Geometry check sheet. Reference: drawing and pictorial views, mm from the part's lowest x, y, z. Give positions to 0.01 mm unless a question says otherwise; leave off trailing zeros. Write each loop counter-clockwise with the first axis right and the second up, starting at its lowest first coordinate (ties: lowest second). Pieces come first, ordered by that corner, then holes. Notation, with made-up numbers: (43, -16.75) - (88, -16.75) arc R28 ccw to (88, 11.25) - close; hole circle Ø5 at (27, 15). An arc over 180 degrees is marked (long way). Write item = value, one per line. Start each with the question number.
(1) Section check A-A, the plane x = 3.5. Enter the section's corners in (y, z).
(2) Section check B-B, the plane z = 6. Enter the section's corners in (x, y).
(3) Section check C-C, the plane y = 1. Enter the section's corners in (x, z).
(4) Thickness scan on L1, parallel to Y at x = 3.5, z = 9; L2, parallel to X at y = 4, z = 33 (1 decimal); L3, parallel to X at y = 4.25, z = 20.5 (1 decimal). Record the ranges inside material, lowest first.
(5) Depth check by flat-ended pin: pin 1 Ø3 at (x, y) = (1.5, 3) entering from -Z; pin 2 Ø1.8 at (x, y) = (3.5, 3.03) entering from +Z. Enter the tip coordinate at first touch or a pass-through.
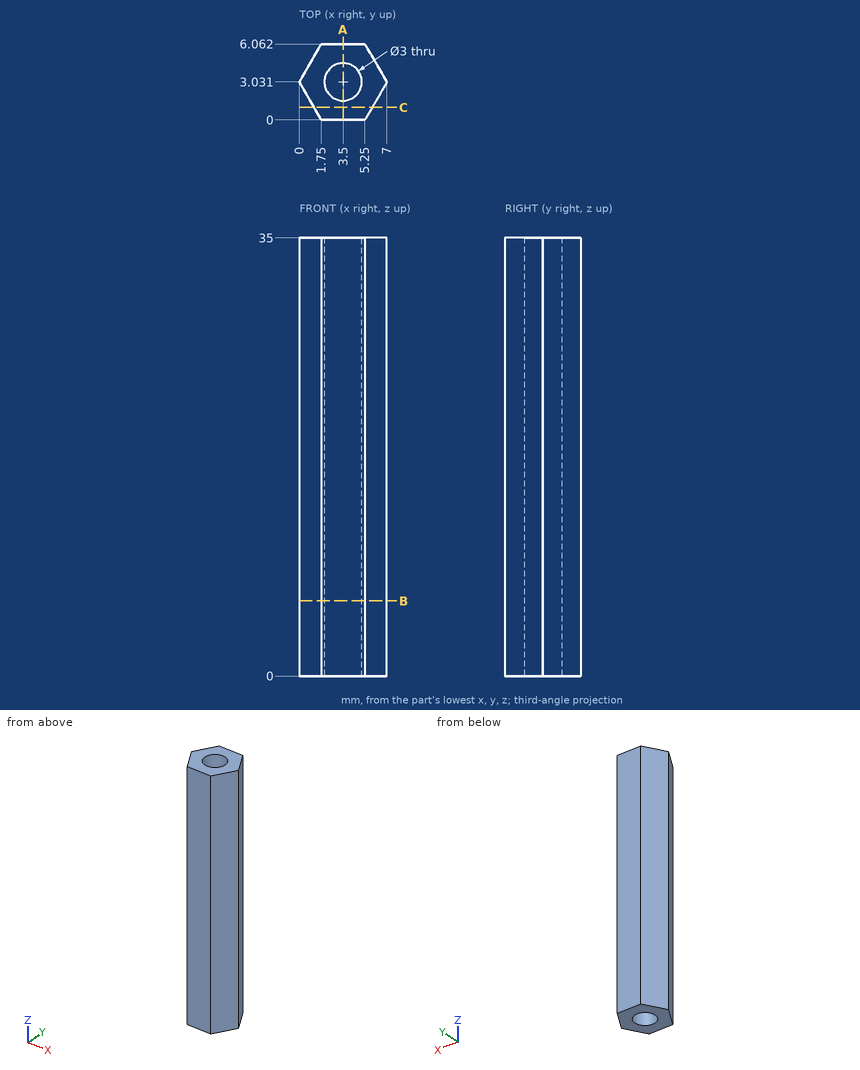
Model answer:
q1.outline = (0, 0) - (1.53, 0) - (1.53, 35) - (0, 35) - close; (4.53, 0) - (6.06, 0) - (6.06, 35) - (4.53, 35) - close
q2.outline = (0, 3.03) - (1.75, 0) - (5.25, 0) - (7, 3.03) - (5.25, 6.06) - (1.75, 6.06) - close; hole circle Ø3 at (3.5, 3.03)
q3.outline = (1.17, 0) - (5.83, 0) - (5.83, 35) - (1.17, 35) - close
q4.L1 = 0 to 1.53, 4.53 to 6.06
q4.L2 = 0.6 to 2.4, 4.6 to 6.4
q4.L3 = 0.7 to 2.6, 4.4 to 6.3
q5.pin_1 = 0
q5.pin_2 = through
